Design review of the part built by this model. Coordinates are the model's own, in mm. Face numbers are marked on the shaded views. A direction names the side the tool comes from. Round coordinates to 2 decimals unless told otherwise and drop trailing zeros. Loops run counter-clockwise (first coordinate to the right, second up) from the corner with the lowest first, then second, coordinate; pieces in that order, holes last. Notation, with made-up numbers: (7, 33.25) - (62, 33.25) arc R8 cw to (62, 40.25) - close; hole circle Ø7 at (-32, -7.5). An arc over 180 degrees is marked (long way). Use one line per item in the form item = value. Start each with the question number.
(1) We need section B-B, the plane x = 0. Write out the cut boundary in (y, z), then the cut area to 3 significant figures.
(2) Machinability: for the marked faces 1, 2 and 3, which of the approach directions +Z, -Z, +X, -X, +Y, -Y give a long, thin tool a straight path to every point of the face, cutting with its end or side? Answer none if there is none.
(3) Wall thickness on probe 1 along Y at (x, z) = (-23.1, 2.25); probe 2 along Y at (x, z) = (0, 3.55); probe 3 along X at (y, z) = (21.3, 3.8): over which ranges is each line inside the solid? List them lowest first. Write a range as [from, to].
(4) We need section A-A, the plane z = 8.75. Write out the cut boundary in (x, y), then the cut area to 3 significant figures.
(5) The part is to be moulded in two halves that separate along Y. For the marked faces 4, 5, 6 and 7, say which applies: released by +Y, released by -Y, zero draft, split by the parting line, or undercut.
(6) For pin 1 (6 mm diameter, centred on x = -26, y = 17, fed in from +Z); pin 2 (14.5 mm diameter, centred on x = -23.1, y = 10, fed in from -Z); pin 3 (1.2 mm diameter, centred on y = 26, z = 8, fed in from +X), all flat-tipped, find the tip position at first contact; note any pin that passes through.
(7) We need section C-C, the plane y = 21.3. Write out the cut boundary in (x, z), then the cut area to 3 significant figures.
(8) We need section D-D, the plane z = 4. Write out the cut boundary in (x, y).
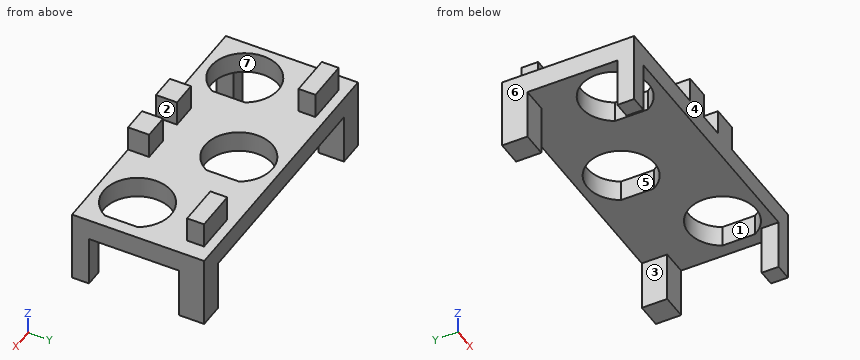
from build123d import *

# Parameters (mm, degrees)
SKETCH_W      = 66.2
SKETCH_H      = 31.3
PAD_DEPTH     = 5
SKETCH001_W   = 10
SKETCH001_H   = 4
SKETCH001_W_2 = 6
SKETCH001_H_2 = 5
PAD001_DEPTH  = 6
SKETCH002_W   = 4
SKETCH002_H   = 4
SKETCH002_W_2 = 6
SKETCH002_H_2 = 6
PAD002_DEPTH  = 12


with BuildPart() as part:
    # Sketch → Pad (new body)
    with BuildSketch(Plane.XY):
        with Locations((0, 15.65)):
            Rectangle(SKETCH_W, SKETCH_H)
        with BuildLine():
            ThreePointArc((-16.1, 13.872983), (-31.1, 10), (-16.1, 6.127017))
            Line((-16.1, 13.872983), (-16.1, 6.127017))
        make_face(mode=Mode.SUBTRACT)
        with BuildLine():
            ThreePointArc((30.1, 13.872983), (15.1, 10), (30.1, 6.127017))
            Line((30.1, 13.872983), (30.1, 6.127017))
        make_face(mode=Mode.SUBTRACT)
        with BuildLine():
            ThreePointArc((7, 25.172983), (-8, 21.3), (7, 17.427017))
            Line((7, 25.172983), (7, 17.427017))
        make_face(mode=Mode.SUBTRACT)
    extrude(amount=PAD_DEPTH)

    # Sketch001 (on Face12 of Pad) → Pad001 (join)
    with BuildSketch(Plane.XY.offset(5)):
        with Locations((24, 27)):
            Rectangle(SKETCH001_W, SKETCH001_H)
        with Locations((6, 2.5)):
            Rectangle(SKETCH001_W_2, SKETCH001_H_2)
    pad001 = extrude(amount=PAD001_DEPTH)

    # Mirrored: Pad001 across Sketch001 V_Axis
    add(pad001.mirror(Plane(origin=(0, 0, 5), x_dir=(0, 0, 1), z_dir=(1, 0, 0))))

    # Sketch002 (on Face3 of Mirrored) → Pad002 (join)
    with BuildSketch(Plane(origin=(0, 0, 0), x_dir=(1, 0, 0), z_dir=(0, 0, -1))):
        with Locations((-31.1, -2)):
            Rectangle(SKETCH002_W, SKETCH002_H)
        with Locations((-30.1, -28.3)):
            Rectangle(SKETCH002_W_2, SKETCH002_H_2)
    pad002 = extrude(amount=PAD002_DEPTH)

    # Mirrored001: Pad002 across Sketch002 V_Axis
    add(pad002.mirror(Plane(origin=(0, 0, 0), x_dir=(0, 0, -1), z_dir=(1, 0, 0))))


solid = part.part
Data:
q1.outline = (0, 0) - (13.3, 0) - (13.3, 5) - (0, 5) - close; (29.3, 0) - (31.3, 0) - (31.3, 5) - (29.3, 5) - close
q1.area = 76.5 mm^2
q2.face_1 = +Z, -Z
q2.face_2 = +Z, +Y, -Y
q2.face_3 = -Z, +Y, -Y
q3.probe_1 = [0, 2], [18, 31.3]
q3.probe_2 = [0, 13.3], [29.3, 31.3]
q3.probe_3 = [-33.1, -8], [7, 33.1]
q4.outline = (-29, 25) - (-19, 25) - (-19, 29) - (-29, 29) - close; (-9, 0) - (-3, 0) - (-3, 5) - (-9, 5) - close; (3, 0) - (9, 0) - (9, 5) - (3, 5) - close; (19, 25) - (29, 25) - (29, 29) - (19, 29) - close
q4.area = 140 mm^2
q5.face_4 = released by -Y
q5.face_5 = undercut
q5.face_6 = zero draft
q5.face_7 = undercut
q6.pin_1 = 5
q6.pin_2 = 0
q6.pin_3 = 29
q7.outline = (-33.1, 0) - (-8, 0) - (-8, 5) - (-33.1, 5) - close; (7, 0) - (33.1, 0) - (33.1, 5) - (7, 5) - close
q7.area = 256 mm^2
q8.outline = (-33.1, 0) - (33.1, 0) - (33.1, 31.3) - (-33.1, 31.3) - close; hole (-16.1, 6.13) - (-16.1, 13.87) arc R8 ccw (long way) to start; hole (7, 17.43) - (7, 25.17) arc R8 ccw (long way) to start; hole (30.1, 6.13) - (30.1, 13.87) arc R8 ccw (long way) to start
